Here's the drawing with two shaded views (mm, measured from the low corner). I have some questions. Round coordinates to 2 decimals unless told otherwise and drop trailing zeros. Loops run counter-clockwise (first coordinate to the right, second up) from the corner with the lowest first, then second, coordinate; pieces in that order, holes last. Notation, with made-up numbers: (-25, -12) - (31, -12) arc R17 cw to (31, 4) - close; hole circle Ø6 at (-8.75, -33.75). An arc over 180 degrees is marked (long way). Answer as CSV lines item,"result".
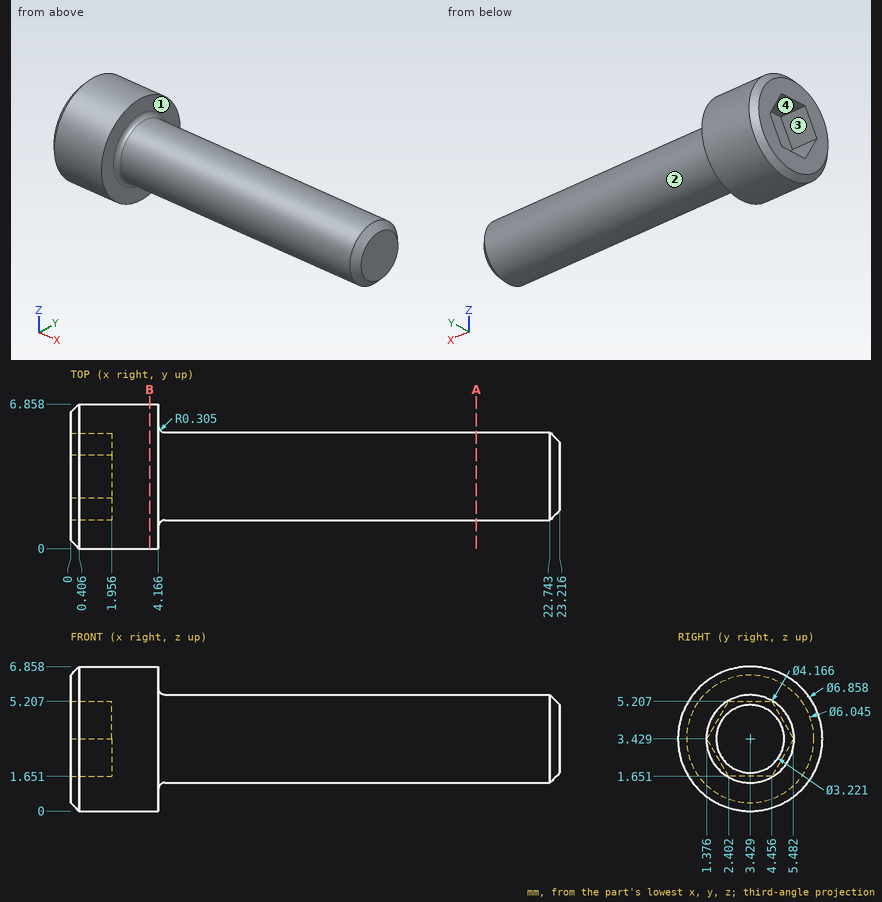
Q1. We'd pull the mould along Y, two halves only. Please class the marked faces 1, 2, 3 and 4: pulls with the +Y half, pulls with the -Y half, needs draft (parallel to the pull), parting line crosses it, or undercut.
Checks:
face 1,"needs draft"
face 2,"parting line crosses it"
face 3,"undercut"
face 4,"undercut"
Q2. Imagine slicing it at A-A (x = 19.25). Write out the boundary of the cut face in (y, z) (1 decimal).
Checks:
outline,"circle Ø4.2 at (3.4, 3.4)"
Q3. Imagine slicing it at B-B (x = 3.75). Write out the boundary of the cut face in (y, z).
Checks:
outline,"circle Ø6.86 at (3.43, 3.43)"
Q4. If I drill on line 1 along X through (y, z) = (1, 3.5) (1 decimal); line 2 along X through (y, z) = (3, 4.25) (1 decimal); line 3 along Y through (x, z) = (19, 3.75), over which ranges is the centre line in solid material (lowest first)? Write a range as [from, to].
Checks:
line 1,"[0, 4.2]"
line 2,"[2, 23.2]"
line 3,"[1.37, 5.49]"
Q5. I'm going to push flat-ended pins straight in: pin 1 Ø1.5 at (x, y) = (2.5, 3) entering from -Z; pin 2 Ø0.6 at (x, y) = (1, 3) entering from +Z; pin 3 Ø1 at (x, y) = (7, 0.5) entering from -Z. Where does each tip first touch, or does it pass through?
Checks:
pin 1,"z = 0"
pin 2,"z = 6.86"
pin 3,"through"
